Could you check a few things on this drawing? It's one solid part, dimensions in mm from its lowest x, y, z. Coordinates: 2 decimals unless noted, no trailing zeros. Order: outer loops, then holes, each group sorted by start corner. A loop starts at its lowest first (then second) coordinate and runs counter-clockwise, first axis right, second up.
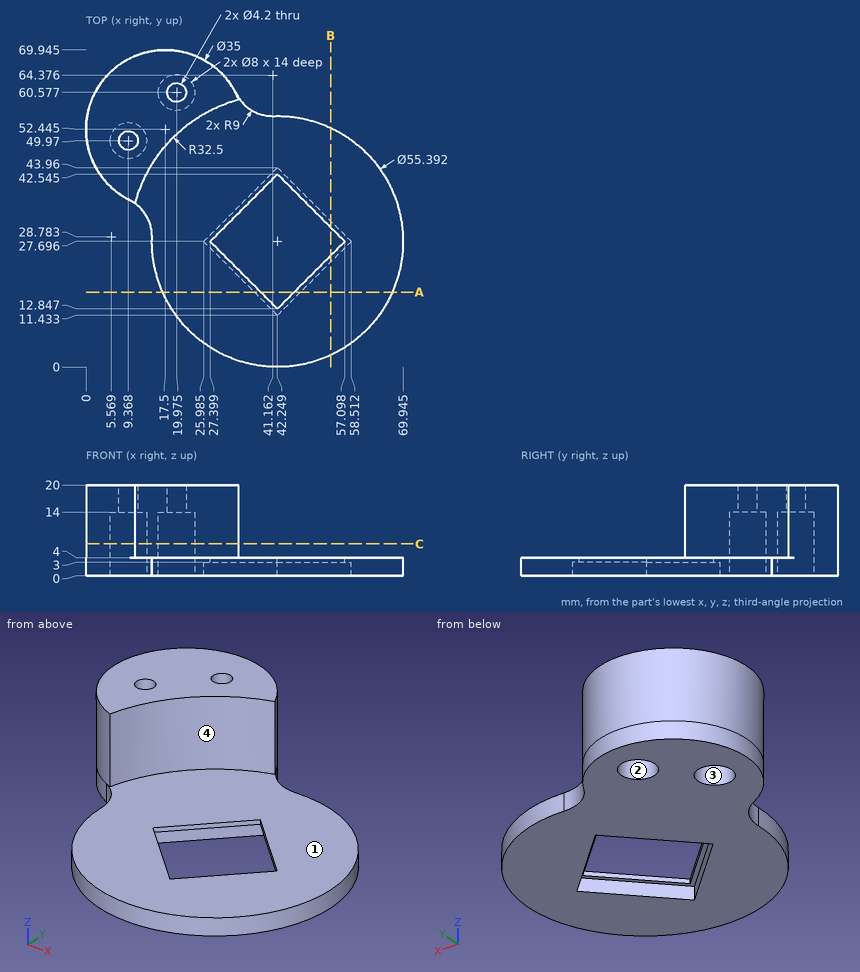
Q1. If we section it at B-B on x = 54: Write out the boundary of the cut face in (y, z) (1 decimal), then the cut area to 3 significant figures.
Q2. I need wall thicknesses on L1, parallel to Y at x = 9.5, z = 16.25 (1 decimal); L2, parallel to Z at x = 59.5, y = 30; L3, parallel to Z at x = 44, y = 13.5. Which ranges of each line are inside material? Lowest first, please.
Q3. If we section it at A-A on y = 16.5: Write out the boundary of the cut face in (x, z) (1 decimal), then the cut area to 3 significant figures.
Q4. We'd pull the mould along Y, two halves only. Please class the marked faces 1, 2, 3 and 4: pulls with the +Y half, pulls with the -Y half, needs draft (parallel to the pull), parting line crosses it, or undercut.
Q5. Will these pins go through, and if not, where does the flat tip stop? pin 1 (1.5 mm diameter, centred on y = 39, z = 12.5, fed in from +X); pin 2 (10 mm diameter, centred on x = 29, y = 38.5, fed in from +Z); pin 3 (2.5 mm diameter, centred on x = 21.5, y = 60.5, fed in from -Z).
Q6. If we section it at C-C on z = 7: Write out the boundary of the cut face in (x, y) (1 decimal).
Reply:
1. outline: (2.6, 0) - (23.2, 0) - (23.2, 3) - (24.6, 3) - (24.6, 4) - (2.6, 4) - close; (30.8, 3) - (32.2, 3) - (32.2, 0) - (52.8, 0) - (52.8, 4) - (30.8, 4) - close
1. area: 167 mm2
2. L1: y = 36.9 to 47.9, 52.1 to 68
2. L2: z = 0 to 4
2. L3: z = 3 to 4
3. outline: (16.9, 0) - (37.2, 0) - (37.2, 3) - (38.6, 3) - (38.6, 4) - (16.9, 4) - close; (45.9, 3) - (47.3, 3) - (47.3, 0) - (67.6, 0) - (67.6, 4) - (45.9, 4) - close
3. area: 165 mm2
4. face 1: needs draft
4. face 2: undercut
4. face 3: undercut
4. face 4: pulls with the -Y half
5. pin 1: stops at x = 12.07
5. pin 2: stops at z = 4
5. pin 3: stops at z = 14
6. outline: (10.9, 36.2) arc R32.5 cw to (33.7, 59.1) arc R17.5 ccw (long way) to start; hole circle Ø8 at (9.4, 50); hole circle Ø8 at (20, 60.6)
